Work out the finished part from the listing and answer in its coordinate system (mm). A direction names the side the tool comes from. Give positions to 0.01 mm unless a question says otherwise; leave off trailing zeros. Order: outer loops, then holes, each group sorted by start corner. A loop starts at its lowest first (then second) coordinate and runs counter-clockwise, first axis right, second up. Notation, with made-up numbers: (43.25, -38) - (90.25, -38) arc R13 ccw to (90.25, -14) - close; hole circle Ø3 at (62.25, -15). An arc over 180 degrees is marked (long way). Write each question's results on one line, items separated by ' | '.
Autodesk Inventor part; units mm, degrees
ref_plane "YZ Plane" through (0, 0, 0) normal (1, 0, 0) x (0, 1, 0)
ref_plane "XZ Plane" through (0, 0, 0) normal (0, 1, 0) x (-1, 0, 0)
ref_plane "XY Plane" through (0, 0, 0) normal (0, 0, 1) x (1, 0, 0)
sketch "Sketch1" plane through (0, 0, 0) normal (0, 0, 1) x (1, 0, 0)
  line L0 (-74.2195, 17.5033) -> (-69.2195, 17.5033)
  line L1 (-69.2195, 17.5033) -> (-69.2195, -62.4967)
  line L2 (-69.2195, -62.4967) -> (-74.2195, -62.4967)
  line L3 (-74.2195, -62.4967) -> (-74.2195, 17.5033)
  line L4 (-69.2195, 17.5033) -> (52.7805, 17.5033)
  line L5 (52.7805, 17.5033) -> (52.7805, 13.4578)
  line L6 (52.7805, 13.4578) -> (-69.2195, 13.4578)
  line L7 (-69.2195, 13.4578) -> (-69.2195, 17.5033)
  line L8 (52.7805, 17.5033) -> (57.7805, 17.5033)
  line L9 (57.7805, 17.5033) -> (57.7805, -62.4967)
  line L10 (57.7805, -62.4967) -> (52.7805, -62.4967)
  line L11 (52.7805, -62.4967) -> (52.7805, 17.5033)
  point P0 (0, 0)
  point P1 (-69.2195, 13.4578)
  dimension "d0" = 5
  dimension "d1" = 80
  dimension "d2" = 122
extrude "Extrusion1" add sketch "Sketch1" along normal blind 5
sketch "Sketch2" plane through (-69.2195, -62.4967, 0) normal (1, 0, 0) x (0, 0, -1)
  point P0 (0, 62.4967)
sketch "Sketch3" plane through (-69.2195, -62.4967, 0) normal (1, 0, 0) x (0, 0, -1)
  point P0 (0, 62.4967)
sketch "Sketch4" plane through (-69.2195, -62.4967, 0) normal (1, 0, 0) x (0, 0, -1)
  line L0 (-5, 73.4545) -> (-4, 73.4545)
  line L1 (-4, 73.4545) -> (-4, 3.4545)
  line L2 (-4, 3.4545) -> (-5, 3.4545)
  line L3 (-5, 3.4545) -> (-5, 73.4545)
  line L4 (-5, 0) -> (-5, 75.9545)
  line L5 (0, 75.9545) -> (-5, 75.9545)
  line L6 (0, 0) -> (-5, 0)
  point P0 (0, 62.4967)
  point P1 (-5, 38.4545)
  dimension "d5" = 1
  dimension "d6" = 70
  dimension "d7" = 2.5
  dimension "d8" = 3.4545
extrude "Extrusion2" add sketch "Sketch4" along normal up to surface (122 mm away)
properties part number "placa" material "PET Plastic"
1. Determine the mould class of faces 4 (the face through (-72, -62.497, 2)), 5 (the face through (57.78, -22, 2)), 6 (the face through (-69.22, -24, 2)) for opening direction X: +X half, -X half, draft (parallel to the pull), parting line (faces both ways), or undercut.
Answer list:
face 4: draft | face 5: +X half | face 6: undercut
2. A cutting plane is placed at B-B, the plane z = 1.8. Write down the section's boundary in (x, y).
Answer list:
outline: (-74.22, -62.5) - (-69.22, -62.5) - (-69.22, 13.46) - (52.78, 13.46) - (52.78, -62.5) - (57.78, -62.5) - (57.78, 17.5) - (-74.22, 17.5) - close
3. A cutting plane is placed at A-A, the plane x = 31.5. Write down the section's boundary in (y, z).
Answer list:
outline: (-59.04, 4) - (10.96, 4) - (10.96, 5) - (-59.04, 5) - close; (13.46, 0) - (17.5, 0) - (17.5, 5) - (13.46, 5) - close
4. A tool of negligible diameter and unlimited length cuts with its end or side. For faces 1 (the face through (55, -62.497, 2)), 2 (the face through (-9, -24, 4)), 3 (the face through (-7, 13.458, 2)), from which of +Z, -Z, +X, -X, +Y, -Y can it reach the whole face along a straight path? Write none if from no direction.
Answer list:
face 1: +Z, -Z, +X, -X, -Y | face 2: -Z, -Y | face 3: +Z, -Z
5. A cutting plane is placed at C-C, the plane y = -47. Write down the section's boundary in (x, z).
Answer list:
outline: (-74.22, 0) - (-69.22, 0) - (-69.22, 4) - (52.78, 4) - (52.78, 0) - (57.78, 0) - (57.78, 5) - (-74.22, 5) - close
6. Straight lines are drawn through the part: line 1 (X direction, y = -37, z = 3.8); line 2 (Y direction, x = -31.5, z = 4.4); line 3 (Y direction, x = 21.5, z = 0.85). For each, find the intervals that lie inside material, in ascending order. Write a range as [from, to].
Answer list:
line 1: [-74.22, -69.22], [52.78, 57.78] | line 2: [-59.04, 10.96], [13.46, 17.5] | line 3: [13.46, 17.5]
7. Given P1, Ø12, axis at x = -40.5, y = -27.5, coming from the -Z side; P2, Ø1, axis at x = -50, z = 4, coming from the -Y side; P3, Ø1, axis at x = 17.5, z = 2, coming from the -Y side, each flat-ended and moving along its own axis, determine where each tip first touches the part or whether it passes through.
Answer list:
P1: z = 4 | P2: y = -59.04 | P3: y = 13.46
